from build123d import *

# Parameters (mm, degrees)
SKETCH_1_W          = 15
SKETCH_1_H          = 15
SKETCH_1_W_2        = 13
SKETCH_1_H_2        = 13
EXTRUDE_1_DEPTH     = 170
SKETCH_2_R          = 1.45
CUT_EXTRUDE_1_DEPTH = 171.825203059
SKETCH_3_R          = 1.45
CUT_EXTRUDE_2_DEPTH = 171.825203059


with BuildPart() as part:
    # 草图1 → 凸台-拉伸1 (new body)
    with BuildSketch(Plane(origin=(0, 0, 0), x_dir=(0, 0, -1), z_dir=(1, 0, 0))):
        Rectangle(SKETCH_1_W, SKETCH_1_H)
        Rectangle(SKETCH_1_W_2, SKETCH_1_H_2, mode=Mode.SUBTRACT)
    extrude(amount=EXTRUDE_1_DEPTH)

    # 草图2 → 切除-拉伸1 (cut, through all)
    with BuildSketch(Plane(origin=(0, 0, -7.5), x_dir=(-1, 0, 0), z_dir=(0, 0, -1))):
        with Locations((-9, 0)):
            Circle(SKETCH_2_R)
        with Locations((-19, 0)):
            Circle(SKETCH_2_R)
        with Locations((-146, 0)):
            Circle(SKETCH_2_R)
        with Locations((-156, 0)):
            Circle(SKETCH_2_R)
    extrude(amount=-CUT_EXTRUDE_1_DEPTH, mode=Mode.SUBTRACT)

    # 草图3 → 切除-拉伸2 (cut, through all)
    with BuildSketch(Plane(origin=(0, 7.5, 0), x_dir=(1, 0, 0), z_dir=(0, 1, 0))):
        with Locations(Location((161, 0, 0), (0, 0, 270))):
            Circle(SKETCH_3_R)
        with Locations(Location((151, 0, 0), (0, 0, 270))):
            Circle(SKETCH_3_R)
        with Locations(Location((24, 0, 0), (0, 0, 270))):
            Circle(SKETCH_3_R)
        with Locations(Location((14, 0, 0), (0, 0, 270))):
            Circle(SKETCH_3_R)
    extrude(amount=-CUT_EXTRUDE_2_DEPTH, mode=Mode.SUBTRACT)


solid = part.part
Work out the finished part from the listing and answer in its coordinate system (mm). A direction names the side the tool comes from. Round coordinates to 2 decimals unless told otherwise and drop trailing zeros. Loops run counter-clockwise (first coordinate to the right, second up) from the corner with the lowest first, then second, coordinate; pieces in that order, holes last. Notation, with made-up numbers: (-18, 16) - (26, 16) arc R14 cw to (26, 23) - close; hole circle Ø4 at (-9.75, 61.25). An arc over 180 degrees is marked (long way). Use one line per item in the form item = value. Start each with the question number.
(1) Find section D-D on x = 24. Determine the outline of the cut face in (y, z).
(2) Consider line 1 (X direction, y = -7.15, z = 0); line 2 (Y direction, x = 94.5, z = 1). Determine where each line is inside the solid, lowest interval first.
(3) Which of the six approach directions +Z, -Z, +X, -X, +Y, -Y give full straight-line access (tool end or side, diameter ignored) to faces 1 (the face through (84, -6.5, 0)), 2 (the face through (154.62, 0.44, 6.99))?
(4) Determine the mould class of faces 3 (the face through (84, 7.5, 0)), 4 (the face through (10.45, 0.06, 6.99)), 5 (the face through (15.438, 7.007, -0.189)) for opening direction Y: +Y half, -Y half, draft (parallel to the pull), parting line (faces both ways), or undercut.
(5) Find section A-A on y = 4.25. Determine the outline of the cut face in (x, z).
(6) Find section B-B on x = 82.5. Determine the outline of the cut face in (y, z), and give its area (3 significant figures).
Answer list:
q1.outline = (-7.5, -7.5) - (7.5, -7.5) - (7.5, -1.45) - (6.5, -1.45) - (6.5, -6.5) - (-6.5, -6.5) - (-6.5, -1.45) - (-7.5, -1.45) - close; (-7.5, 1.45) - (-6.5, 1.45) - (-6.5, 6.5) - (6.5, 6.5) - (6.5, 1.45) - (7.5, 1.45) - (7.5, 7.5) - (-7.5, 7.5) - close
q2.line_1 = 0 to 12.55, 15.45 to 22.55, 25.45 to 149.55, 152.45 to 159.55, 162.45 to 170
q2.line_2 = -7.5 to -6.5, 6.5 to 7.5
q3.face_1 = +X, -X
q3.face_2 = +Z, -Z
q4.face_3 = +Y half
q4.face_4 = undercut
q4.face_5 = draft
q5.outline = (0, -7.5) - (170, -7.5) - (170, -6.5) - (0, -6.5) - close; (0, 6.5) - (170, 6.5) - (170, 7.5) - (0, 7.5) - close
q6.outline = (-7.5, -7.5) - (7.5, -7.5) - (7.5, 7.5) - (-7.5, 7.5) - close; hole (-6.5, -6.5) - (6.5, -6.5) - (6.5, 6.5) - (-6.5, 6.5) - close
q6.area = 56.0 mm^2
